Check sheet for the modelled part. Datum: model origin and axes. Units: mm. Give positions to 0.01 mm unless a question says otherwise; leave off trailing zeros. Use one line per item in the form item = value.
from build123d import *

# Parameters (mm, degrees)
F1_W     = 122.6013228297
F1_H     = 65.9010410309
F1_W_2   = 2.7029693592
F1_H_2   = 25.326666655
F1_H_3   = 17.8375145576
F2_DEPTH = 25


with BuildPart() as f2:
    # F1 (on face) → F2 (new body)
    with BuildSketch(Plane.XZ):
        with Locations((61.3006614149, 32.9505205154)):
            Rectangle(F1_W, F1_H)
        with BuildLine():
            Line((39.001939275, 31.5462090075), (36.9968463977, 31.5462090075))
            Line((36.9968463977, 31.5462090075), (36.4604189526, 34.0877293299))
            Line((36.4604189526, 34.0877293299), (36.3302181164, 34.0877293299))
            add(Edge.make_bspline(
                [(36.3302181164, 34.0877293299), (34.9969615539, 32.4107425598), (33.6715170415, 31.81442273)],
                knots=[0, 0, 0, 1, 1, 1], degree=2))
            add(Edge.make_bspline(
                [(33.6715170415, 31.81442273), (32.3460725291, 31.2181029003), (30.3566037522, 31.2181029003)],
                knots=[0, 0, 0, 1, 1, 1], degree=2))
            add(Edge.make_bspline(
                [(30.3566037522, 31.2181029003), (27.7057147274, 31.2181029003), (26.2005930611, 32.587815697)],
                knots=[0, 0, 0, 1, 1, 1], degree=2))
            add(Edge.make_bspline(
                [(26.2005930611, 32.587815697), (24.6954713948, 33.9575284937), (24.6954713948, 36.4782166823)],
                knots=[0, 0, 0, 1, 1, 1], degree=2))
            add(Edge.make_bspline(
                [(24.6954713948, 36.4782166823), (24.6954713948, 41.8789473673), (33.3355988842, 42.1393490396)],
                knots=[0, 0, 0, 1, 1, 1], degree=2))
            Line((33.3355988842, 42.1393490396), (36.3614663171, 42.2383016751))
            Line((36.3614663171, 42.2383016751), (36.3614663171, 43.3476127995))
            add(Edge.make_bspline(
                [(36.3614663171, 43.3476127995), (36.3614663171, 45.4464502788), (35.4604765307, 46.4463927007)],
                knots=[0, 0, 0, 1, 1, 1], degree=2))
            add(Edge.make_bspline(
                [(35.4604765307, 46.4463927007), (34.5594867443, 47.4463351226), (32.5700179674, 47.4463351226)],
                knots=[0, 0, 0, 1, 1, 1], degree=2))
            add(Edge.make_bspline(
                [(32.5700179674, 47.4463351226), (30.3409796519, 47.4463351226), (27.5286415902, 46.0818303594)],
                knots=[0, 0, 0, 1, 1, 1], degree=2))
            Line((27.5286415902, 46.0818303594), (26.6953562386, 48.149419638))
            add(Edge.make_bspline(
                [(26.6953562386, 48.149419638), (28.0129887008, 48.8629202203), (29.5832107853, 49.2691468292)],
                knots=[0, 0, 0, 1, 1, 1], degree=2))
            add(Edge.make_bspline(
                [(29.5832107853, 49.2691468292), (31.1534328697, 49.6753734381), (32.7366750377, 49.6753734381)],
                knots=[0, 0, 0, 1, 1, 1], degree=2))
            add(Edge.make_bspline(
                [(32.7366750377, 49.6753734381), (35.9239915075, 49.6753734381), (37.4629653913, 48.2613923571)],
                knots=[0, 0, 0, 1, 1, 1], degree=2))
            add(Edge.make_bspline(
                [(37.4629653913, 48.2613923571), (39.001939275, 46.8474112762), (39.001939275, 43.7225912077)],
                knots=[0, 0, 0, 1, 1, 1], degree=2))
            Line((39.001939275, 43.7225912077), (39.001939275, 31.5462090075))
        make_face(mode=Mode.SUBTRACT)
        with BuildLine():
            Line((60.0580185031, 31.5462090075), (56.9019502339, 31.5462090075))
            Line((56.9019502339, 31.5462090075), (50.1315067522, 49.3837235651))
            Line((50.1315067522, 49.3837235651), (53.027173349, 49.3837235651))
            Line((53.027173349, 49.3837235651), (56.8707020332, 38.8062076333))
            add(Edge.make_bspline(
                [(56.8707020332, 38.8062076333), (58.1727103951, 35.0928797852), (58.4018638668, 33.9887766944)],
                knots=[0, 0, 0, 1, 1, 1], degree=2))
            Line((58.4018638668, 33.9887766944), (58.532064703, 33.9887766944))
            add(Edge.make_bspline(
                [(58.532064703, 33.9887766944), (58.7091378402, 34.8481022132), (59.6622079611, 37.5588836226)],
                knots=[0, 0, 0, 1, 1, 1], degree=2))
            add(Edge.make_bspline(
                [(59.6622079611, 37.5588836226), (60.615278082, 40.269665032), (63.932795388, 49.3837235651)],
                knots=[0, 0, 0, 1, 1, 1], degree=2))
            Line((63.932795388, 49.3837235651), (66.8284619848, 49.3837235651))
            Line((66.8284619848, 49.3837235651), (60.0580185031, 31.5462090075))
        make_face(mode=Mode.SUBTRACT)
        with Locations((45.9156036765, 44.209542335)):
            Rectangle(F1_W_2, F1_H_2, mode=Mode.SUBTRACT)
        with Locations((71.0443650605, 40.4649662863)):
            Rectangle(F1_W_2, F1_H_3, mode=Mode.SUBTRACT)
        with BuildLine():
            Line((93.0352862924, 31.5462090075), (90.3323169332, 31.5462090075))
            Line((90.3323169332, 31.5462090075), (90.3323169332, 43.0872111271))
            add(Edge.make_bspline(
                [(90.3323169332, 43.0872111271), (90.3323169332, 45.2641691081), (89.3401865615, 46.339628015)],
                knots=[0, 0, 0, 1, 1, 1], degree=2))
            add(Edge.make_bspline(
                [(89.3401865615, 46.339628015), (88.3480561897, 47.4150869219), (86.2283865766, 47.4150869219)],
                knots=[0, 0, 0, 1, 1, 1], degree=2))
            add(Edge.make_bspline(
                [(86.2283865766, 47.4150869219), (83.4316726153, 47.4150869219), (82.1296642534, 45.9021532054)],
                knots=[0, 0, 0, 1, 1, 1], degree=2))
            add(Edge.make_bspline(
                [(82.1296642534, 45.9021532054), (80.8276558916, 44.3892194889), (80.8276558916, 40.9050451126)],
                knots=[0, 0, 0, 1, 1, 1], degree=2))
            Line((80.8276558916, 40.9050451126), (80.8276558916, 31.5462090075))
            Line((80.8276558916, 31.5462090075), (78.1246865323, 31.5462090075))
            Line((78.1246865323, 31.5462090075), (78.1246865323, 49.3837235651))
            Line((78.1246865323, 49.3837235651), (80.3224766472, 49.3837235651))
            Line((80.3224766472, 49.3837235651), (80.7599514568, 46.9411558782))
            Line((80.7599514568, 46.9411558782), (80.8901522929, 46.9411558782))
            add(Edge.make_bspline(
                [(80.8901522929, 46.9411558782), (81.7234376445, 48.2587883404), (83.2207472607, 48.9853090063)],
                knots=[0, 0, 0, 1, 1, 1], degree=2))
            add(Edge.make_bspline(
                [(83.2207472607, 48.9853090063), (84.7180568768, 49.7118296723), (86.5564926838, 49.7118296723)],
                knots=[0, 0, 0, 1, 1, 1], degree=2))
            add(Edge.make_bspline(
                [(86.5564926838, 49.7118296723), (89.7802653878, 49.7118296723), (91.4077758401, 48.1572316882)],
                knots=[0, 0, 0, 1, 1, 1], degree=2))
            add(Edge.make_bspline(
                [(91.4077758401, 48.1572316882), (93.0352862924, 46.6026337041), (93.0352862924, 43.1809557291)],
                knots=[0, 0, 0, 1, 1, 1], degree=2))
            Line((93.0352862924, 43.1809557291), (93.0352862924, 31.5462090075))
        make_face(mode=Mode.SUBTRACT)
        with BuildLine():
            add(Edge.make_bspline(
                [(69.9194298359, 52.8574818745), (69.4637269092, 53.305372751), (69.4637269092, 54.2167786043)],
                knots=[0, 0, 0, 1, 1, 1], degree=2))
            add(Edge.make_bspline(
                [(69.4637269092, 54.2167786043), (69.4637269092, 55.143808558), (69.9194298359, 55.5760753341)],
                knots=[0, 0, 0, 1, 1, 1], degree=2))
            add(Edge.make_bspline(
                [(69.9194298359, 55.5760753341), (70.3751327625, 56.0083421102), (71.0625931776, 56.0083421102)],
                knots=[0, 0, 0, 1, 1, 1], degree=2))
            add(Edge.make_bspline(
                [(71.0625931776, 56.0083421102), (71.7135973585, 56.0083421102), (72.1849243855, 55.5682632839)],
                knots=[0, 0, 0, 1, 1, 1], degree=2))
            add(Edge.make_bspline(
                [(72.1849243855, 55.5682632839), (72.6562514125, 55.1281844576), (72.6562514125, 54.2167786043)],
                knots=[0, 0, 0, 1, 1, 1], degree=2))
            add(Edge.make_bspline(
                [(72.6562514125, 54.2167786043), (72.6562514125, 53.305372751), (72.1849243855, 52.8574818745)],
                knots=[0, 0, 0, 1, 1, 1], degree=2))
            add(Edge.make_bspline(
                [(72.1849243855, 52.8574818745), (71.7135973585, 52.409590998), (71.0625931776, 52.409590998)],
                knots=[0, 0, 0, 1, 1, 1], degree=2))
            add(Edge.make_bspline(
                [(71.0625931776, 52.409590998), (70.3751327625, 52.409590998), (69.9194298359, 52.8574818745)],
                knots=[0, 0, 0, 1, 1, 1], degree=2))
        make_face(mode=Mode.SUBTRACT)
    extrude(amount=F2_DEPTH)


solid = f2.part
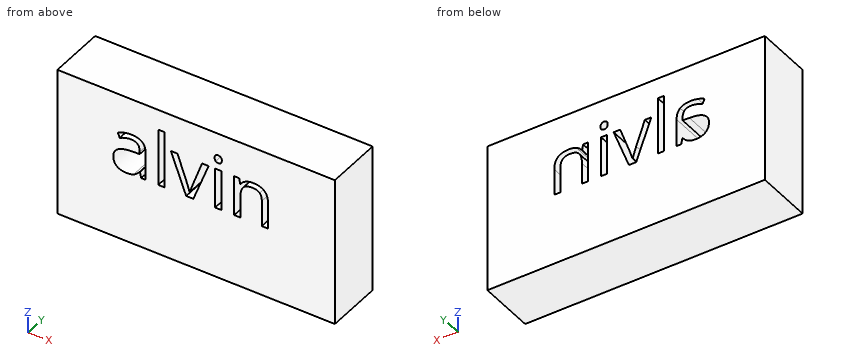
Item 1: Gauge pin test, flat end, axial feed: P1, Ø6, axis at x = 29, z = 40.5, coming from the -Y side. Record the tip position at first contact, or that the pin passes through.
Answer block:
P1 = -25
Item 2: Thickness scan on L1, parallel to X at y = -13.5, z = 54.5; L2, parallel to Z at x = 92, y = -4.25; L3, parallel to X at y = -4.5, z = 53. Record the ranges inside material, lowest first.
Answer block:
L1 = 0 to 44.56, 47.27 to 69.48, 72.64 to 122.6
L2 = 0 to 31.55, 47.45 to 65.9
L3 = 0 to 44.56, 47.27 to 69.79, 72.31 to 122.6
Item 3: Section check A-A on y = -17.25. Give the number of separate pieces and of enclosed holes in the cut face, then the cut area to 3 significant figures.
Answer block:
separate_pieces = 1
enclosed_holes = 6
area = 7,570 mm2
